from build123d import *

# Parameters (mm, degrees)
SKETCH_1_R          = 40
SKETCH_1_R_2        = 3.1
EXTRUDE_2_DEPTH     = 5
SKETCH_2_R          = 0.75
CUT_EXTRUDE_1_DEPTH = 5


with BuildPart() as part:
    # 草图1 → 凸台-拉伸2 (new body)
    # profile 1 of 11: a face of its own
    with BuildSketch(Plane.XY):
        with Locations((48.296474355, 27.924907455)):
            Circle(SKETCH_1_R)
        with BuildLine():
            Line((81.82316003, 10.300317263), (81.07316003, 9.001279158))
            Line((81.07316003, 9.001279158), (80.32316003, 7.702241052))
            Line((80.32316003, 7.702241052), (79.12969775, 8.391286821))
            ThreePointArc((79.12969775, 8.391286821), (48.296474355, -8.575092545), (17.46325096, 8.391286821))
            Line((17.46325096, 8.391286821), (16.26978868, 7.702241052))
            Line((16.26978868, 7.702241052), (15.51978868, 9.001279158))
            Line((15.51978868, 9.001279158), (14.76978868, 10.300317263))
            Line((14.76978868, 10.300317263), (15.96325096, 10.989363032))
            ThreePointArc((15.96325096, 10.989363032), (16.69953266, 46.197380619), (46.84834221, 64.396168926))
            Line((46.84834221, 64.396168926), (46.84834221, 66.091480515))
            Line((46.84834221, 66.091480515), (49.787930978, 66.091480515))
            Line((49.787930978, 66.091480515), (49.787930978, 64.394422905))
            ThreePointArc((49.787930978, 64.394422905), (74.627902029, 53.201495766), (84.796474355, 27.924907455))
            ThreePointArc((84.796474355, 27.924907455), (83.739475455, 19.204605107), (80.62969775, 10.989363032))
            Line((80.62969775, 10.989363032), (81.82316003, 10.300317263))
        make_face(mode=Mode.SUBTRACT)
    # profile 2 of 11: a face of its own
    with BuildSketch(Plane.XY):
        with BuildLine():
            Line((52.565394479, 27.19229608), (54.167021201, 26.267596461))
            ThreePointArc((54.167021201, 26.267596461), (54.338838783, 27.088347762), (54.396474355, 27.924907455))
            ThreePointArc((54.396474355, 27.924907455), (53.108328748, 31.67404833), (49.787930978, 33.839766468))
            Line((49.787930978, 33.839766468), (49.787930978, 32.638782116))
            Line((49.787930978, 32.638782116), (46.84834221, 32.638782116))
            Line((46.84834221, 32.638782116), (46.84834221, 33.850522469))
            ThreePointArc((46.84834221, 33.850522469), (43.027133101, 30.998023585), (42.425927509, 26.267596461))
            Line((42.425927509, 26.267596461), (43.927397053, 27.134470306))
            Line((43.927397053, 27.134470306), (45.427397053, 24.536394095))
            Line((45.427397053, 24.536394095), (43.925927509, 23.66952025))
            ThreePointArc((43.925927509, 23.66952025), (48.296474355, 21.824907455), (52.667021201, 23.66952025))
            Line((52.667021201, 23.66952025), (51.065394479, 24.594219869))
            Line((51.065394479, 24.594219869), (52.565394479, 27.19229608))
        make_face()
        with Locations((48.296474355, 27.924907455)):
            Circle(SKETCH_1_R_2, mode=Mode.SUBTRACT)
    # profile 3 of 11: a face of its own
    with BuildSketch(Plane.XY):
        with BuildLine():
            ThreePointArc((15.96325096, 10.989363032), (16.686547117, 9.674907455), (17.46325096, 8.391286821))
            Line((17.46325096, 8.391286821), (43.925927509, 23.66952025))
            ThreePointArc((43.925927509, 23.66952025), (43.013719392, 24.874907455), (42.425927509, 26.267596461))
            Line((42.425927509, 26.267596461), (15.96325096, 10.989363032))
        make_face()
    # profile 4 of 11: a face of its own
    with BuildSketch(Plane.XY):
        with BuildLine():
            Line((16.26978868, 7.702241052), (17.46325096, 8.391286821))
            ThreePointArc((17.46325096, 8.391286821), (16.686547117, 9.674907455), (15.96325096, 10.989363032))
            Line((15.96325096, 10.989363032), (14.76978868, 10.300317263))
            Line((14.76978868, 10.300317263), (15.51978868, 9.001279158))
            Line((15.51978868, 9.001279158), (16.26978868, 7.702241052))
        make_face()
    # profile 5 of 11: a face of its own
    with BuildSketch(Plane.XY):
        with BuildLine():
            ThreePointArc((52.667021201, 23.66952025), (53.579229318, 24.874907455), (54.167021201, 26.267596461))
            Line((54.167021201, 26.267596461), (52.565394479, 27.19229608))
            Line((52.565394479, 27.19229608), (51.065394479, 24.594219869))
            Line((51.065394479, 24.594219869), (52.667021201, 23.66952025))
        make_face()
    # profile 6 of 11: a face of its own
    with BuildSketch(Plane.XY):
        with BuildLine():
            Line((49.787930978, 32.638782116), (49.787930978, 33.839766468))
            ThreePointArc((49.787930978, 33.839766468), (48.3187942, 34.024866621), (46.84834221, 33.850522469))
            Line((46.84834221, 33.850522469), (46.84834221, 32.638782116))
            Line((46.84834221, 32.638782116), (49.787930978, 32.638782116))
        make_face()
    # profile 7 of 11: a face of its own
    with BuildSketch(Plane.XY):
        with BuildLine():
            ThreePointArc((42.425927509, 26.267596461), (43.013719392, 24.874907455), (43.925927509, 23.66952025))
            Line((43.925927509, 23.66952025), (45.427397053, 24.536394095))
            Line((45.427397053, 24.536394095), (43.927397053, 27.134470306))
            Line((43.927397053, 27.134470306), (42.425927509, 26.267596461))
        make_face()
    # profile 8 of 11: a face of its own
    with BuildSketch(Plane.XY):
        with BuildLine():
            Line((49.787930978, 33.839766468), (49.787930978, 64.394422905))
            ThreePointArc((49.787930978, 64.394422905), (48.318154178, 64.424901017), (46.84834221, 64.396168926))
            Line((46.84834221, 64.396168926), (46.84834221, 33.850522469))
            ThreePointArc((46.84834221, 33.850522469), (48.3187942, 34.024866621), (49.787930978, 33.839766468))
        make_face()
    # profile 9 of 11: a face of its own
    with BuildSketch(Plane.XY):
        with BuildLine():
            ThreePointArc((46.84834221, 64.396168926), (48.318154178, 64.424901017), (49.787930978, 64.394422905))
            Line((49.787930978, 64.394422905), (49.787930978, 66.091480515))
            Line((49.787930978, 66.091480515), (46.84834221, 66.091480515))
            Line((46.84834221, 66.091480515), (46.84834221, 64.396168926))
        make_face()
    # profile 10 of 11: a face of its own
    with BuildSketch(Plane.XY):
        with BuildLine():
            Line((80.32316003, 7.702241052), (81.07316003, 9.001279158))
            Line((81.07316003, 9.001279158), (81.82316003, 10.300317263))
            Line((81.82316003, 10.300317263), (80.62969775, 10.989363032))
            ThreePointArc((80.62969775, 10.989363032), (79.906401593, 9.674907455), (79.12969775, 8.391286821))
            Line((79.12969775, 8.391286821), (80.32316003, 7.702241052))
        make_face()
    # profile 11 of 11: a face of its own
    with BuildSketch(Plane.XY):
        with BuildLine():
            ThreePointArc((79.12969775, 8.391286821), (79.906401593, 9.674907455), (80.62969775, 10.989363032))
            Line((80.62969775, 10.989363032), (54.167021201, 26.267596461))
            ThreePointArc((54.167021201, 26.267596461), (53.579229318, 24.874907455), (52.667021201, 23.66952025))
            Line((52.667021201, 23.66952025), (79.12969775, 8.391286821))
        make_face()
    extrude(amount=EXTRUDE_2_DEPTH)

    # 草图2 → 切除-拉伸1 (cut)
    with BuildSketch(Plane.XY.offset(5)):
        with Locations((14.954496309, 47.174907455)):
            Circle(SKETCH_2_R)
        with Locations((81.638452401, 47.174907455)):
            Circle(SKETCH_2_R)
        with Locations((48.296474355, -10.575092545)):
            Circle(SKETCH_2_R)
    extrude(amount=-CUT_EXTRUDE_1_DEPTH, mode=Mode.SUBTRACT)


solid = part.part
Verification items for the finished model (mm, model axes). A direction names the side the tool comes from. Round coordinates to 2 decimals unless told otherwise and drop trailing zeros. Loops run counter-clockwise (first coordinate to the right, second up) from the corner with the lowest first, then second, coordinate; pieces in that order, holes last. Notation, with made-up numbers: (53.25, -3) - (81.25, -3) arc R19 ccw to (81.25, 32) - close; hole circle Ø10 at (39, -39). An arc over 180 degrees is marked (long way). Answer in a Markdown table with one row per item. Add a question column.
Q1. Gauge pin test, flat ends, axial feed: pin 1 (1 mm diameter, centred on x = 18.5, z = 4, fed in from +Y); pin 2 (1.5 mm diameter, centred on y = 54, z = 1.5, fed in from -X); pin 3 (1.5 mm diameter, centred on x = 25.5, z = 2.5, fed in from +Y). Record the tip position at first contact, or that the pin passes through.
Q2. Tool access check on faces 1 (the face through (43.062, 31.057, 2.465)), 2 (the face through (51, 25, 0)). Record the directions out of +Z, -Z, +X, -X, +Y, -Y that give a thin tool (end or side, any length) a straight path to the whole face; none if there is none.
Q3. Material ranges on line 1 (Y direction, x = 59, z = 2.8); line 2 (X direction, y = 52, z = 3.35); line 3 (X direction, y = 56, z = 4.5), recorded low to high.
Q4. Section check B-B on x = 19.5. Enter the section's corners in (y, z).
Q5. Release check for a two-part mould opening along Y. For faces 3 (the face through (51, 25, 5)), 4 (the face through (8.335, 29.684, 2.465)), 5 (the face through (48.81, -8.57, 2.46)), 6 (the face through (16.445, 45.75, 2.465)) record: pulls with the +Y half, pulls with the -Y half, needs draft (parallel to the pull), parting line crosses it, or undercut.
Q6. Section check D-D on z = 3.65. Enter the section's corners in (x, y).
Q7. Section check A-A on y = 12. Enter the section's corners in (x, z).
Q8. Section check C-C on y = 40. Enter the section's corners in (x, z).
Found:
| question | item | result |
|---|---|---|
| 1 | pin 1 | stops at y = 55.16 |
| 1 | pin 2 | stops at x = 17.33 |
| 1 | pin 3 | stops at y = 61.3 |
| 2 | face 1 | +Z, -Z |
| 2 | face 2 | -Z, +X, -X, +Y, -Y |
| 3 | line 1 | y = -10.62 to -6.97, 20.01 to 23.48, 62.82 to 66.47 |
| 3 | line 2 | x = 16.35 to 20.86, 46.85 to 49.79, 75.73 to 80.24 |
| 3 | line 3 | x = 19.8 to 24.97, 46.85 to 49.79, 71.62 to 76.79 |
| 4 | outline | (0.16, 0) - (5.5, 0) - (5.5, 5) - (0.16, 5) - close; (9.57, 0) - (13.03, 0) - (13.03, 5) - (9.57, 5) - close; (50.35, 0) - (55.69, 0) - (55.69, 5) - (50.35, 5) - close |
| 5 | face 3 | needs draft |
| 5 | face 4 | parting line crosses it |
| 5 | face 5 | undercut |
| 5 | face 6 | undercut |
| 6 | outline | circle Ø80 at (48.3, 27.92); hole circle Ø1.5 at (14.95, 47.17); hole (15.96, 10.99) - (42.43, 26.27) arc R6.1 cw to (46.85, 33.85) - (46.85, 64.4) arc R36.5 ccw to start; hole (17.46, 8.39) arc R36.5 ccw to (79.13, 8.39) - (52.67, 23.67) arc R6.1 cw to (43.93, 23.67) - close; hole circle Ø6.2 at (48.3, 27.92); hole circle Ø1.5 at (48.3, -10.58); hole (49.79, 33.84) arc R6.1 cw to (54.17, 26.27) - (80.63, 10.99) arc R36.5 ccw to (49.79, 64.39) - close; hole circle Ø1.5 at (81.64, 47.17) |
| 7 | outline | (11.6, 0) - (15.45, 0) - (15.45, 5) - (11.6, 5) - close; (17.71, 0) - (23.71, 0) - (23.71, 5) - (17.71, 5) - close; (72.88, 0) - (78.88, 0) - (78.88, 5) - (72.88, 5) - close; (81.14, 0) - (84.99, 0) - (84.99, 5) - (81.14, 5) - close |
| 8 | outline | (10.16, 0) - (13.85, 0) - (13.85, 5) - (10.16, 5) - close; (46.85, 0) - (49.79, 0) - (49.79, 5) - (46.85, 5) - close; (82.74, 0) - (86.43, 0) - (86.43, 5) - (82.74, 5) - close |
